CAD build for the part. Positions are in the model's coordinates, mm. Coordinates: 2 decimals unless noted, no trailing zeros. Write each loop counter-clockwise with the first axis right and the second up, starting at its lowest first coordinate (ties: lowest second). Pieces come first, ordered by that corner, then holes. Notation, with made-up numbers: (89, -8) - (100, -8) arc R19 cw to (100, 25) - close; hole circle Ø4 at (6.5, -20.75). An arc over 180 degrees is marked (long way). Answer in a Markdown table with one row per item. Add a question column.
Q1. Drill centre lines: line 1 along X through (y, z) = (50, 6.25); line 2 along X through (y, z) = (34.5, 11.75); line 3 along Y through (x, z) = (176.5, 12.25). Where is each one in solid material? Low to high. Write a range as from..to.
Q2. Two-plate mould, pull along X, no slides. Class faces 1 (the cylindrical face through (177.693, 45.494, 8.112)), 2 (the flat face through (0, 49, 8)), 3 (the flat face through (164, 100, 8)): +X half, -X half, draft (parallel to the pull), parting line (faces both ways), or undercut.
Q3. Pin check, flat tip, straight feed: pin 1 (1.5 mm diameter, centred on x = 123.5, z = 7, fed in from -Y). Stop position of the tip, or through.
Q4. Band-saw the part on C-C (y = 42). List the corners of the cut face in (x, z), and give its area (3 significant figures).
Q5. Band-saw the part on A-A (x = 192). List the corners of the cut face in (y, z).
Q6. Band-saw the part on B-B (z = 7). State how many separate pieces and enclosed holes the cut face has, and give its area (3 significant figures).
```python
from build123d import *

# Parameters (mm, degrees)
F0_W     = 332
F0_H     = 100
F1_DEPTH = 16
F3_DEPTH = 25
F5_DEPTH = 25


with BuildPart() as f1:
    # F0 (on Top) → F1 (new body)
    with BuildSketch(Plane.XY):
        with Locations((166, 50)):
            Rectangle(F0_W, F0_H)
    extrude(amount=F1_DEPTH)

    # F2 (on face) → F3 (cut)
    with BuildSketch(Plane.XY.offset(16)):
        with BuildLine():
            Line((125, 50), (140, 50))
            Line((140, 50), (155, 50))
            ThreePointArc((155, 50), (140, 65), (125, 50))
        make_face()
        with BuildLine():
            Line((140, 50), (140, 35))
            ThreePointArc((140, 35), (150.6066017178, 39.3933982822), (155, 50))
            Line((155, 50), (140, 50))
        make_face()
        with BuildLine():
            ThreePointArc((125, 50), (129.3933982822, 39.3933982822), (140, 35))
            Line((140, 35), (140, 50))
            Line((140, 50), (125, 50))
        make_face()
        with BuildLine():
            ThreePointArc((126, 65.5), (123.4393398282, 66.5606601718), (124.5, 64))
            Line((124.5, 64), (124.5, 65.5))
            Line((124.5, 65.5), (126, 65.5))
        make_face()
        with BuildLine():
            Line((124.5, 65.5), (124.5, 64))
            ThreePointArc((124.5, 64), (125.5606601718, 64.4393398282), (126, 65.5))
            Line((126, 65.5), (124.5, 65.5))
        make_face()
        with BuildLine():
            ThreePointArc((124.5, 36), (123.4393398282, 33.4393398282), (126, 34.5))
            Line((126, 34.5), (124.5, 34.5))
            Line((124.5, 34.5), (124.5, 36))
        make_face()
        with BuildLine():
            Line((124.5, 34.5), (126, 34.5))
            ThreePointArc((126, 34.5), (125.5606601718, 35.5606601718), (124.5, 36))
            Line((124.5, 36), (124.5, 34.5))
        make_face()
        with BuildLine():
            Line((155.5, 34.5), (154, 34.5))
            ThreePointArc((154, 34.5), (155.5, 33), (157, 34.5))
            ThreePointArc((157, 34.5), (156.5606601718, 35.5606601718), (155.5, 36))
            Line((155.5, 36), (155.5, 34.5))
        make_face()
        with BuildLine():
            ThreePointArc((155.5, 36), (154.4393398282, 35.5606601718), (154, 34.5))
            Line((154, 34.5), (155.5, 34.5))
            Line((155.5, 34.5), (155.5, 36))
        make_face()
        with BuildLine():
            Line((155.5, 65.5), (155.5, 64))
            ThreePointArc((155.5, 64), (156.5606601718, 64.4393398282), (157, 65.5))
            ThreePointArc((157, 65.5), (155.5, 67), (154, 65.5))
            Line((154, 65.5), (155.5, 65.5))
        make_face()
        with BuildLine():
            ThreePointArc((154, 65.5), (154.4393398282, 64.4393398282), (155.5, 64))
            Line((155.5, 64), (155.5, 65.5))
            Line((155.5, 65.5), (154, 65.5))
        make_face()
        with BuildLine():
            Line((192, 50), (192, 35))
            ThreePointArc((192, 35), (202.6066017178, 39.3933982822), (207, 50))
            Line((207, 50), (192, 50))
        make_face()
        with BuildLine():
            Line((177, 50), (192, 50))
            Line((192, 50), (207, 50))
            ThreePointArc((207, 50), (192, 65), (177, 50))
        make_face()
        with BuildLine():
            ThreePointArc((177, 50), (181.3933982822, 39.3933982822), (192, 35))
            Line((192, 35), (192, 50))
            Line((192, 50), (177, 50))
        make_face()
        with BuildLine():
            ThreePointArc((178, 65.5), (175.4393398282, 66.5606601718), (176.5, 64))
            Line((176.5, 64), (176.5, 65.5))
            Line((176.5, 65.5), (178, 65.5))
        make_face()
        with BuildLine():
            Line((176.5, 65.5), (176.5, 64))
            ThreePointArc((176.5, 64), (177.5606601718, 64.4393398282), (178, 65.5))
            Line((178, 65.5), (176.5, 65.5))
        make_face()
        with BuildLine():
            ThreePointArc((176.5, 36), (175.4393398282, 33.4393398282), (178, 34.5))
            Line((178, 34.5), (176.5, 34.5))
            Line((176.5, 34.5), (176.5, 36))
        make_face()
        with BuildLine():
            Line((176.5, 34.5), (178, 34.5))
            ThreePointArc((178, 34.5), (177.5606601718, 35.5606601718), (176.5, 36))
            Line((176.5, 36), (176.5, 34.5))
        make_face()
        with BuildLine():
            ThreePointArc((207.5, 36), (206.4393398282, 35.5606601718), (206, 34.5))
            Line((206, 34.5), (207.5, 34.5))
            Line((207.5, 34.5), (207.5, 36))
        make_face()
        with BuildLine():
            Line((207.5, 34.5), (206, 34.5))
            ThreePointArc((206, 34.5), (207.5, 33), (209, 34.5))
            ThreePointArc((209, 34.5), (208.5606601718, 35.5606601718), (207.5, 36))
            Line((207.5, 36), (207.5, 34.5))
        make_face()
        with BuildLine():
            Line((207.5, 65.5), (207.5, 64))
            ThreePointArc((207.5, 64), (208.5606601718, 64.4393398282), (209, 65.5))
            ThreePointArc((209, 65.5), (207.5, 67), (206, 65.5))
            Line((206, 65.5), (207.5, 65.5))
        make_face()
        with BuildLine():
            ThreePointArc((206, 65.5), (206.4393398282, 64.4393398282), (207.5, 64))
            Line((207.5, 64), (207.5, 65.5))
            Line((207.5, 65.5), (206, 65.5))
        make_face()
    extrude(amount=-F3_DEPTH, mode=Mode.SUBTRACT)

    # F4 (on face) → F5 (cut)
    with BuildSketch(Plane.XY.offset(16)):
        with BuildLine():
            ThreePointArc((51.6347899064, 50), (44.8063627817, 52.8284271247), (47.6347899064, 46))
            ThreePointArc((47.6347899064, 46), (50.4632170312, 47.1715728753), (51.6347899064, 50))
        make_face()
        with BuildLine():
            ThreePointArc((286, 50), (279.1715728753, 52.8284271247), (282, 46))
            ThreePointArc((282, 46), (284.8284271247, 47.1715728753), (286, 50))
        make_face()
    extrude(amount=-F5_DEPTH, mode=Mode.SUBTRACT)


solid = f1.part
```
Checked values:
| question | item | result |
|---|---|---|
| 1 | line 1 | x = 0..43.63, 51.63..125, 155..177, 207..278, 286..332 |
| 1 | line 2 | x = 0..123, 126..154, 157..175, 178..206, 209..332 |
| 1 | line 3 | y = 0..33, 36..64, 67..100 |
| 2 | face 1 | undercut |
| 2 | face 2 | -X half |
| 2 | face 3 | draft |
| 3 | pin 1 | stops at y = 0 |
| 4 | outline | (0, 0) - (127.31, 0) - (127.31, 16) - (0, 16) - close; (152.69, 0) - (179.31, 0) - (179.31, 16) - (152.69, 16) - close; (204.69, 0) - (332, 0) - (332, 16) - (204.69, 16) - close |
| 4 | area | 4,500 mm² |
| 5 | outline | (0, 0) - (35, 0) - (35, 16) - (0, 16) - close; (65, 0) - (100, 0) - (100, 16) - (65, 16) - close |
| 6 | separate pieces | 1 |
| 6 | enclosed holes | 12 |
| 6 | area | 31,600 mm² |
